Check sheet for the modelled part. Datum: model origin and axes. Units: mm. Face numbers are marked on the shaded views. Coordinates: 2 decimals unless noted, no trailing zeros. Write each loop counter-clockwise with the first axis right and the second up, starting at its lowest first coordinate (ties: lowest second). Pieces come first, ordered by that corner, then holes. Notation, with made-up numbers: (-29, 40) - (3, 40) arc R27 cw to (3, 72) - close; hole circle Ø7 at (-9, -27.5). An arc over 180 degrees is marked (long way). Answer as CSV lines item,"result". Start each with the question number.
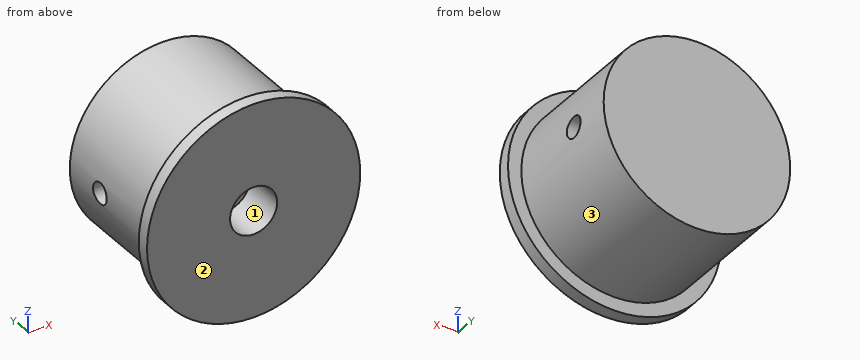
from build123d import *


with BuildPart() as part:
    # Sketch1 → Revolve1 (revolve)
    with BuildSketch(Plane(origin=(0, 0, 0), x_dir=(0, 0, -1), z_dir=(1, 0, 0)), mode=Mode.PRIVATE) as revolve1_sk:
        Polygon((-12.7, 0), (-12.7, 1.5), (-11.1125, 1.5), (-11.1125, 16.5), (0, 16.5), (0, 5), (-2.8067, 5), (-2.8067, 0), align=None)
    revolve(revolve1_sk.sketch.rotate(Axis((0, -1000, 0), (0, 1, 0)), 180), axis=Axis((0, -1000, 0), (0, 1, 0)))

    # Sketch4 → M3x0.5 Tapped Hole1 (revolve, cut)
    with BuildSketch(Plane(origin=(11.1125, 11.025, 0), x_dir=(0, 0, -1), z_dir=(0, 1, 0))):
        Polygon((0, 0), (0, 10.751075774), (1.25, 10), (1.25, 0), align=None)
    m3x0_5_tapped_hole1 = revolve(axis=Axis((17.4625, 11.025, 0), (-1, 0, 0)), mode=Mode.SUBTRACT)

    # Mirror1: M3x0.5 Tapped Hole1 across plane
    add(m3x0_5_tapped_hole1.mirror(Plane(origin=(0, 0, 0), x_dir=(0, 0, 1), z_dir=(1, 0, 0))), mode=Mode.SUBTRACT)


solid = part.part
(1) Material ranges on probe 1 along X at (y, z) = (2.7, 0); probe 2 along Z at (x, y) = (2.5, 10.25); probe 3 along Z at (x, y) = (-0.5, 4), recorded low to high. Write a range as from..to.
(2) Cross-section at D-D on y = 7.75. Record the boundary of the cut face in (x, z) (1 decimal).
(3) Cross-section at B-B on x = 0. Record the boundary of the cut face in (y, z), plus the area to 3 significant figures.
(4) Release check for a two-part mould opening along X. For the marked faces 1, 2 and 3 record: pulls with the +X half, pulls with the -X half, needs draft (parallel to the pull), parting line crosses it, or undercut.
(5) Cross-section at A-A on y = 4. Record the boundary of the cut face in (x, z) (1 decimal), plus the area to 3 significant figures.
(6) Cross-section at C-C on z = 4.5. Record the boundary of the cut face in (x, y), plus the area to 3 significant figures.
(7) Go/stop test with flat-tipped pins: P1, Ø1, axis at y = 9.5, z = 6, coming from the -X side; P2, Ø2, axis at y = 7.5, z = -2, coming from the -X side; P3, Ø2, axis at y = 11.025, z = 0, coming from the -X side. Record where each tip stops, or that it passes through.
Checked values:
1,probe 1,"-11.11..-2.81, 2.81..11.11"
1,probe 2,"-10.83..-0.98, 0.98..10.83"
1,probe 3,"-11.1..-2.76, 2.76..11.1"
2,outline,"circle Ø22.2 at (0, 0)"
3,outline,"(0, -12.7) - (1.5, -12.7) - (1.5, -11.11) - (16.5, -11.11) - (16.5, 11.11) - (1.5, 11.11) - (1.5, 12.7) - (0, 12.7) - (0, 2.81) - (5, 2.81) - (5, -2.81) - (0, -2.81) - close"
3,area,"343 mm^2"
4,face 1,"undercut"
4,face 2,"needs draft"
4,face 3,"parting line crosses it"
5,outline,"circle Ø22.2 at (0, 0); hole circle Ø5.6 at (0, 0)"
5,area,"363 mm^2"
6,outline,"(-11.88, 0) - (11.88, 0) - (11.88, 1.5) - (10.16, 1.5) - (10.16, 16.5) - (-10.16, 16.5) - (-10.16, 1.5) - (-11.88, 1.5) - close"
6,area,"340 mm^2"
7,P1,"x = -9.66"
7,P2,"x = -11.07"
7,P3,"x = -0.96"
